```python
from build123d import *

# Parameters (mm, degrees)
SKETCH1_R                                           = 2.1
BOSS_EXTRUDE1_DEPTH                                 = 4.5
SKETCH2_R                                           = 15.5
CUT_EXTRUDE1_DEPTH                                  = 1
SKETCH3_W                                           = 12.5
SKETCH3_H                                           = 6
CUT_EXTRUDE2_DEPTH                                  = 1
SKETCH4_R                                           = 1.6
CUT_EXTRUDE3_DEPTH                                  = 5.5
CSK_FOR_M4_COUNTERSUNK_FLAT_HEAD_SCREW1_D           = 3.2
CSK_FOR_M4_COUNTERSUNK_FLAT_HEAD_SCREW1_CSINK_D     = 5.8
CSK_FOR_M4_COUNTERSUNK_FLAT_HEAD_SCREW1_CSINK_ANGLE = 90


with BuildPart() as part:
    # Sketch1 → Boss-Extrude1 (new body)
    with BuildSketch(Plane(origin=(0, 0, 0), x_dir=(1, 0, 0), z_dir=(0, 1, 0))):
        with BuildLine():
            Line((11.5, -19.918584287), (0, 0))
            Line((0, 0), (-11.5, -19.918584287))
            Line((-11.5, -19.918584287), (-19.5, -33.774990748))
            ThreePointArc((-19.5, -33.774990748), (0, -39), (19.5, -33.774990748))
            Line((19.5, -33.774990748), (11.5, -19.918584287))
        make_face()
        with Locations((-10.42932356, -32.098157425)):
            Circle(SKETCH1_R, mode=Mode.SUBTRACT)
        with Locations((10.42932356, -32.098157425)):
            Circle(SKETCH1_R, mode=Mode.SUBTRACT)
        Polygon((11.5, 19.918584287), (0, 0), (11.5, -19.918584287), align=None)
        with BuildLine():
            Line((-11.5, 19.918584287), (0, 0))
            Line((0, 0), (11.5, 19.918584287))
            Line((11.5, 19.918584287), (19.5, 33.774990748))
            ThreePointArc((19.5, 33.774990748), (0, 39), (-19.5, 33.774990748))
            Line((-19.5, 33.774990748), (-11.5, 19.918584287))
        make_face()
        with Locations((-10.42932356, 32.098157425)):
            Circle(SKETCH1_R, mode=Mode.SUBTRACT)
        with Locations((10.42932356, 32.098157425)):
            Circle(SKETCH1_R, mode=Mode.SUBTRACT)
        Polygon((-11.5, -19.918584287), (0, 0), (-11.5, 19.918584287), align=None)
    extrude(amount=BOSS_EXTRUDE1_DEPTH)

    # Sketch2 → Cut-Extrude1 (cut)
    with BuildSketch(Plane(origin=(0, 4.5, 0), x_dir=(1, 0, 0), z_dir=(0, 1, 0))):
        Circle(SKETCH2_R)
    extrude(amount=-CUT_EXTRUDE1_DEPTH, mode=Mode.SUBTRACT)

    # Sketch3 → Cut-Extrude2 (cut)
    with BuildSketch(Plane(origin=(0, 3.5, 0), x_dir=(1, 0, 0), z_dir=(0, 1, 0))):
        with Locations((5.25, 0)):
            Rectangle(SKETCH3_W, SKETCH3_H)
    extrude(amount=-CUT_EXTRUDE2_DEPTH, mode=Mode.SUBTRACT)

    # Sketch4 → Cut-Extrude3 (cut, through all)
    with BuildSketch(Plane(origin=(0, 4.5, 0), x_dir=(1, 0, 0), z_dir=(0, 1, 0))):
        with Locations((-4.5, -18.5)):
            Circle(SKETCH4_R)
        with Locations((2.5, -18.5)):
            Circle(SKETCH4_R)
        with Locations((-4.5, 18.5)):
            Circle(SKETCH4_R)
        with Locations((2.5, 18.5)):
            Circle(SKETCH4_R)
    extrude(amount=-CUT_EXTRUDE3_DEPTH, mode=Mode.SUBTRACT)

    # CSK for M4 Countersunk Flat Head Screw1 (through all)
    with Locations(Plane(origin=(-4.5, 4.5, 18.5), x_dir=(0, 0, 1), z_dir=(0, 1, 0))):
        with Locations((0, 0), (0, 7), (-37, 0), (-37, 7)):
            CounterSinkHole(CSK_FOR_M4_COUNTERSUNK_FLAT_HEAD_SCREW1_D / 2, CSK_FOR_M4_COUNTERSUNK_FLAT_HEAD_SCREW1_CSINK_D / 2, counter_sink_angle=CSK_FOR_M4_COUNTERSUNK_FLAT_HEAD_SCREW1_CSINK_ANGLE)


solid = part.part
```
Read the model definition and answer for the solid it produces. Units are mm, in the model's axes. A direction names the side the tool comes from. Coordinates: 2 decimals unless noted, no trailing zeros. Loops run counter-clockwise (first coordinate to the right, second up) from the corner with the lowest first, then second, coordinate; pieces in that order, holes last.
(1) The part is cut by section A-A (z = 18.5). Determine the outline of the cut face in (x, y).
Solution:
outline: (-11.5, 0) - (-6.1, 0) - (-6.1, 3.2) - (-7.4, 4.5) - (-11.5, 4.5) - close; (-2.9, 0) - (0.9, 0) - (0.9, 3.2) - (-0.4, 4.5) - (-1.6, 4.5) - (-2.9, 3.2) - close; (4.1, 0) - (11.5, 0) - (11.5, 4.5) - (5.4, 4.5) - (4.1, 3.2) - close
(2) The part is cut by section B-B (x = 2.5). Determine the outline of the cut face in (y, z), and give its area (3 significant figures).
Solution:
outline: (0, -38.92) - (4.5, -38.92) - (4.5, -21.4) - (3.2, -20.1) - (0, -20.1) - close; (0, -16.9) - (3.2, -16.9) - (4.5, -15.6) - (4.5, -15.3) - (3.5, -15.3) - (3.5, -3) - (2.5, -3) - (2.5, 3) - (3.5, 3) - (3.5, 15.3) - (4.5, 15.3) - (4.5, 15.6) - (3.2, 16.9) - (0, 16.9) - close; (0, 20.1) - (3.2, 20.1) - (4.5, 21.4) - (4.5, 38.92) - (0, 38.92) - close
area: 282 mm2
(3) The mould has two halves that part along Z. Classify faces 1 (the face through (0, 2, -39)), 2 (the face through (0, 4.5, 28)), 3 (the face through (-4.708, 1.622, 16.914)): released by +Z, released by -Z, zero draft, split by the parting line, or undercut.
Solution:
face 1: released by -Z
face 2: zero draft
face 3: undercut
(4) A tool of negligible diameter and unlimited length cuts with its end or side. For faces 4 (the face through (15.556, 2.218, 26.944)), 5 (the face through (-0.2, 4, 15.5)), 6 (the face through (-15.444, 2.218, 26.75)), 7 (the face through (5, 2.5, 0)), from which of +Z, -Z, +X, -X, +Y, -Y can it reach the whole face along a straight path? Write none if from no direction.
Solution:
face 4: +X, +Y, -Y
face 5: +Y
face 6: -X, +Y, -Y
face 7: +X, +Y
(5) Consider line 1 along X through (y, z) = (2, 18.5); line 2 along X through (y, z) = (0.55, -19.5); line 3 along Z through (x, y) = (3, 3.35). Determine where each line is inside the solid, lowest interval first.
Solution:
line 1: x = -11.5 to -6.1, -2.9 to 0.9, 4.1 to 11.5
line 2: x = -11.5 to -5.75, -3.25 to 1.25, 3.75 to 11.5
line 3: z = -38.88 to -20.18, -16.82 to -3, 3 to 16.82, 20.18 to 38.88
(6) The part is cut by section D-D (x = -13.5). Determine the outline of the cut face in (y, z).
Solution:
outline: (0, -36.59) - (4.5, -36.59) - (4.5, -23.38) - (0, -23.38) - close; (0, 23.38) - (4.5, 23.38) - (4.5, 36.59) - (0, 36.59) - close
(7) Flat-ended cylindrical pins translate along their axes: pin 1 Ø2 at (y, z) = (1.5, -10.5) entering from -X; pin 2 Ø0.8 at (x, y) = (6, 3) entering from +Z; pin 3 Ø1 at (y, z) = (1.5, -8) entering from +X; pin 4 Ø3.5 at (x, z) = (10.43, -32.1) entering from +Y. Find the tip coordinate at first contact, or state that the pin passes through.
Solution:
pin 1: stops at x = -11.5
pin 2: stops at z = 38.6
pin 3: stops at x = 11.5
pin 4: passes through
(8) The part is cut by section C-C (y = 1.15). Count the separate pieces of the cut face and the enclosed holes in it, and give its area (3 significant figures).
Solution:
separate pieces: 1
enclosed holes: 8
area: 1,960 mm2
